Check sheet for the modelled part. Datum: model origin and axes. Units: mm. A direction names the side the tool comes from. Give positions to 0.01 mm unless a question says otherwise; leave off trailing zeros. Write each loop counter-clockwise with the first axis right and the second up, starting at its lowest first coordinate (ties: lowest second). Pieces come first, ordered by that corner, then holes. Notation, with made-up numbers: (-33.75, 44.5) -> (24.25, 44.5) arc R13 cw to (24.25, 67.5) -> close; hole circle Ø3 at (66, -17.75). An arc over 180 degrees is marked (long way). Answer as a JSON object with one key per item and string values.
from build123d import *

# Parameters (mm, degrees)
SKETCH1_R                                        = 47.625
BOSS_EXTRUDE1_DEPTH                              = 14.2875
SKETCH2_R                                        = 12.7
CUT_EXTRUDE1_DEPTH                               = 69.850663804
BOSS_EXTRUDE2_START                              = 3.175
SKETCH3_R                                        = 15.875
SKETCH3_R_2                                      = 12.7
BOSS_EXTRUDE2_DEPTH                              = 3.175
CBORE_FOR_3_8_SOCKET_HEAD_CAP_SCREW1_D           = 10.0838
CBORE_FOR_3_8_SOCKET_HEAD_CAP_SCREW1_CBORE_D     = 15.875
CBORE_FOR_3_8_SOCKET_HEAD_CAP_SCREW1_CBORE_DEPTH = 9.525
F_5_16_18_TAPPED_HOLE1_D                         = 6.5278


with BuildPart() as part:
    # Sketch1 → Boss-Extrude1 (new body)
    with BuildSketch(Plane.XY):
        Circle(SKETCH1_R)
    extrude(amount=BOSS_EXTRUDE1_DEPTH)

    # Sketch2 → Cut-Extrude1 (cut, through all)
    with BuildSketch(Plane.XY.offset(14.2875)):
        Circle(SKETCH2_R)
    extrude(amount=-CUT_EXTRUDE1_DEPTH, mode=Mode.SUBTRACT)

    # Sketch3 → Boss-Extrude2 (add)
    with BuildSketch(Plane.XY.offset(14.2875).offset(BOSS_EXTRUDE2_START)):
        Circle(SKETCH3_R)
        Circle(SKETCH3_R_2, mode=Mode.SUBTRACT)
    extrude(amount=-BOSS_EXTRUDE2_DEPTH)

    # CBORE for 3/8 Socket Head Cap Screw1 (through all)
    with Locations(Plane.XY.offset(14.2875)):
        with Locations((0, -33.3375), (-31.705846612, -10.30185405), (-19.595290848, 26.97060405), (19.595290848, 26.97060405), (31.705846612, -10.30185405), (0, 0)):
            CounterBoreHole(CBORE_FOR_3_8_SOCKET_HEAD_CAP_SCREW1_D / 2, CBORE_FOR_3_8_SOCKET_HEAD_CAP_SCREW1_CBORE_D / 2, CBORE_FOR_3_8_SOCKET_HEAD_CAP_SCREW1_CBORE_DEPTH)

    # 5/16-18 Tapped Hole1 (through all)
    with Locations(Plane.XY.offset(14.2875)):
        with Locations((-19.595290848, -26.97060405), (-31.705846612, 10.30185405), (0, 33.3375), (31.705846612, 10.30185405), (19.595290848, -26.97060405), (0, 0)):
            Hole(F_5_16_18_TAPPED_HOLE1_D / 2)


solid = part.part
1. Sectioned sample at A-A, the plane y = 0. Enter the section's corners in (x, z) (1 decimal).
Determined:
{"outline": "(-47.6, 0) -> (-12.7, 0) -> (-12.7, 17.5) -> (-15.9, 17.5) -> (-15.9, 14.3) -> (-47.6, 14.3) -> close; (12.7, 0) -> (47.6, 0) -> (47.6, 14.3) -> (15.9, 14.3) -> (15.9, 17.5) -> (12.7, 17.5) -> close"}
2. Sectioned sample at B-B, the plane x = 0. Enter the section's corners in (y, z) (1 decimal), plus the area to 3 significant figures.
Determined:
{"outline": "(-47.6, 0) -> (-38.4, 0) -> (-38.4, 4.8) -> (-41.3, 4.8) -> (-41.3, 14.3) -> (-47.6, 14.3) -> close; (-28.3, 0) -> (-12.7, 0) -> (-12.7, 17.5) -> (-15.9, 17.5) -> (-15.9, 14.3) -> (-25.4, 14.3) -> (-25.4, 4.8) -> (-28.3, 4.8) -> close; (12.7, 0) -> (30.1, 0) -> (30.1, 14.3) -> (15.9, 14.3) -> (15.9, 17.5) -> (12.7, 17.5) -> close; (36.6, 0) -> (47.6, 0) -> (47.6, 14.3) -> (36.6, 14.3) -> close", "area": "726 mm^2"}
3. Access from +Z, -Z, +X, -X, +Y, -Y to the whole of each face (thin tool, end or side, straight path). Record for faces 4 (the face through (-39.636, -9.953, 9.592)), 5 (the face through (-21.922, 22.498, 2.348)).
Determined:
{"face 4": "+Z", "face 5": "+Z, -Z"}
4. Sectioned sample at C-C, the plane x = 32.5. Enter the section's corners in (y, z).
Determined:
{"outline": "(-34.81, 0) -> (-15.28, 0) -> (-15.28, 4.76) -> (-18.2, 4.76) -> (-18.2, 14.29) -> (-34.81, 14.29) -> close; (-5.32, 0) -> (7.14, 0) -> (7.14, 14.29) -> (-2.4, 14.29) -> (-2.4, 4.76) -> (-5.32, 4.76) -> close; (13.47, 0) -> (34.81, 0) -> (34.81, 14.29) -> (13.47, 14.29) -> close"}
5. Sectioned sample at D-D, the plane z = 11. State how many separate pieces and enclosed holes the cut face has, plus the area to 3 significant figures.
Determined:
{"separate pieces": "1", "enclosed holes": "11", "area": "5,460 mm^2"}
6. Mould release check, pull along X, two halves, no side actions. Record for faces 1 (the face through (0.71, 30.15, 7.04)), 2 (the face through (-7, 11, 17.462)), 3 (the face through (-3.441, -15.497, 15.897)): released by +X, released by -X, zero draft, split by the parting line, or undercut.
Determined:
{"face 1": "undercut", "face 2": "zero draft", "face 3": "split by the parting line"}
7. Scan lines: L1, parallel to X at y = 30.5, z = 1; L2, parallel to Y at x = -32, z = 1; L3, parallel to X at y = -6, z = 14.25. Record each from-to range of solid material in increasing order. Write a range as [from, to].
Determined:
{"L1": "[-36.58, -23.2], [-15.99, -1.61], [1.61, 15.99], [23.2, 36.58]", "L2": "[-35.27, -15.34], [-5.27, 7.05], [13.55, 35.27]", "L3": "[-47.25, -38.38], [-25.04, -11.19], [11.19, 25.04], [38.38, 47.25]"}
8. Go/stop test with flat-tipped pins: P1, Ø2, axis at x = -28, z = 8, coming from the +Y side; P2, Ø14.5, axis at x = -19.6, y = 26.97, coming from the -Z side; P3, Ø4, axis at y = 37.5, z = 15.5, coming from the +X side; P4, Ø2, axis at x = 30.5, z = 15, coming from the -Y side. Record where each tip stops, or that it passes through.
Determined:
{"P1": "y = 39.23", "P2": "z = 0", "P3": "x = 31.28", "P4": "y = -37.15"}
